```python
from build123d import *

# Parameters (mm, degrees)
CROQUIS1_R                                           = 20
SALIENTE_EXTRUIR1_DEPTH                              = 7
REFRENTADO_PARA_TORNILLO_TAP_N_CON_CABEZ_D           = 3.4
REFRENTADO_PARA_TORNILLO_TAP_N_CON_CABEZ_CSINK_D     = 6.72
REFRENTADO_PARA_TORNILLO_TAP_N_CON_CABEZ_CSINK_ANGLE = 90
TALADRO_DE_MARGEN_PARA_M31_D                         = 3.4
CROQUIS8_R                                           = 5
CORTAR_EXTRUIR1_DEPTH                                = 3
CROQUIS9_R                                           = 7
SALIENTE_EXTRUIR2_DEPTH                              = 25


with BuildPart() as part:
    # Croquis1 → Saliente-Extruir1 (new body)
    with BuildSketch(Plane.XY):
        Circle(CROQUIS1_R)
    extrude(amount=SALIENTE_EXTRUIR1_DEPTH)

    # Refrentado para tornillo tapón con cabeza plana de clavija de M31 (through all)
    with Locations(Plane.XY.offset(7)):
        with Locations((0, 15.5), (15.5, 0), (0, -15.5), (-15.5, 0)):
            CounterSinkHole(REFRENTADO_PARA_TORNILLO_TAP_N_CON_CABEZ_D / 2, REFRENTADO_PARA_TORNILLO_TAP_N_CON_CABEZ_CSINK_D / 2, counter_sink_angle=REFRENTADO_PARA_TORNILLO_TAP_N_CON_CABEZ_CSINK_ANGLE)

    # Taladro de margen para M31 (through all)
    with Locations(Plane.XY.offset(7)):
        with Locations((0, 0)):
            Hole(TALADRO_DE_MARGEN_PARA_M31_D / 2)

    # Croquis8 → Cortar-Extruir1 (cut)
    with BuildSketch(Plane(origin=(0, 0, 0), x_dir=(-1, 0, 0), z_dir=(0, 0, -1))):
        Circle(CROQUIS8_R)
    extrude(amount=-CORTAR_EXTRUIR1_DEPTH, mode=Mode.SUBTRACT)

    # Croquis9 → Saliente-Extruir2 (add)
    with BuildSketch(Plane.XY.offset(7)):
        Circle(CROQUIS9_R)
    extrude(amount=SALIENTE_EXTRUIR2_DEPTH)


solid = part.part
```
Work out the finished part from the listing and answer in its coordinate system (mm). A direction names the side the tool comes from. Give positions to 0.01 mm unless a question says otherwise; leave off trailing zeros. Write each loop counter-clockwise with the first axis right and the second up, starting at its lowest first coordinate (ties: lowest second). Pieces come first, ordered by that corner, then holes.
(1) The mould has two halves that part along X. Classify faces 4 (the cylindrical face through (0.37, 13.84, 2.63)), 5 (the cylindrical face through (6.466, -2.681, 19.325)), 6 (the flat face through (0, 0, 32)): pulls with the +X half, pulls with the -X half, needs draft (parallel to the pull), parting line crosses it, or undercut.
Final values:
face 4: undercut
face 5: parting line crosses it
face 6: needs draft
(2) Flat-ended cylindrical pins translate along their axes: pin 1 Ø6 at (x, z) = (2, 21.5) entering from -Y; pin 2 Ø3 at (x, z) = (3.5, 17) entering from -Y; pin 3 Ø4 at (y, z) = (-11, 5) entering from +X; pin 4 Ø4 at (x, y) = (0, 15.5) entering from -Z. Find the tip coordinate at first contact, or state that the pin passes through.
Final values:
pin 1: stops at y = -7
pin 2: stops at y = -6.71
pin 3: stops at x = 17.86
pin 4: stops at z = 0
(3) The part is cut by section C-C on y = -15.5. Write down the section's boundary in (x, z).
Final values:
outline: (-12.64, 0) - (-1.7, 0) - (-1.7, 5.34) - (-3.36, 7) - (-12.64, 7) - close; (1.7, 0) - (12.64, 0) - (12.64, 7) - (3.36, 7) - (1.7, 5.34) - close
(4) Straight lines are drawn through the part: line 1 (Y direction, x = 0, z = 2); line 2 (Y direction, x = 0, z = 4.6); line 3 (Z direction, x = -2.5, y = 3.5). For each, find the intervals that lie inside material, in ascending order.
Final values:
line 1: y = -20 to -17.2, -13.8 to -5, 5 to 13.8, 17.2 to 20
line 2: y = -20 to -17.2, -13.8 to -1.7, 1.7 to 13.8, 17.2 to 20
line 3: z = 3 to 32
(5) The part is cut by section A-A on y = 0. Write down the section's boundary in (x, z), plus the area to 3 significant figures.
Final values:
outline: (-20, 0) - (-17.2, 0) - (-17.2, 5.34) - (-18.86, 7) - (-20, 7) - close; (-13.8, 0) - (-5, 0) - (-5, 3) - (-1.7, 3) - (-1.7, 7) - (1.7, 7) - (1.7, 3) - (5, 3) - (5, 0) - (13.8, 0) - (13.8, 5.34) - (12.14, 7) - (7, 7) - (7, 32) - (-7, 32) - (-7, 7) - (-12.14, 7) - (-13.8, 5.34) - close; (17.2, 0) - (20, 0) - (20, 7) - (18.86, 7) - (17.2, 5.34) - close
area: 533 mm2
(6) Which of the six approach directions +Z, -Z, +X, -X, +Y, -Y give full straight-line access (tool end or side, diameter ignored) to faces 1 (the flat face through (0, -9, 7)), 2 (the flat face through (0, 0, 7)), 3 (the cylindrical face through (0.221, -13.814, 2.633))?
Final values:
face 1: +Z
face 2: -Z
face 3: +Z, -Z
